Here's the drawing with two shaded views (mm, measured from the low corner). I have some questions. Round coordinates to 2 decimals unless told otherwise and drop trailing zeros. Write each loop counter-clockwise with the first axis right and the second up, starting at its lowest first coordinate (ties: lowest second). Pieces come first, ordered by that corner, then holes. Notation, with made-up numbers: M -26.75,36 L 17.25,36 A17 cw 17.25,58 Z; hole C -40,88.25 d10. An arc over 180 degrees is marked long. Write item = value, one per line. Start each with the question number.
(1) I want a section at A-A (y = 165). List the corners of the cut face in (x, z) for me, and give its area (3 significant figures).
(2) Will these pins go through, and if not, where does the flat tip stop? pin 1 Ø14.5 at (x, y) = (121, 165) entering from -Z; pin 2 Ø3 at (x, z) = (112.5, 4) entering from +Y; pin 3 Ø3 at (y, z) = (51.5, 3.5) entering from +X.
(3) I want a section at B-B (x = 91.5). List the corners of the cut face in (y, z) for me.
(4) I want a section at D-D (x = 121). List the corners of the cut face in (y, z) for me.
(5) I want a section at C-C (z = 1.9). List the corners of the cut face in (x, y) for me.
(6) I need wall thicknesses on line 1 along X through (y, z) = (225, 2.1); line 2 along Y through (x, z) = (121, 4.4); line 3 along Y through (x, z) = (72.5, 2.2). Which ranges of each line are inside material? Lowest first, please.
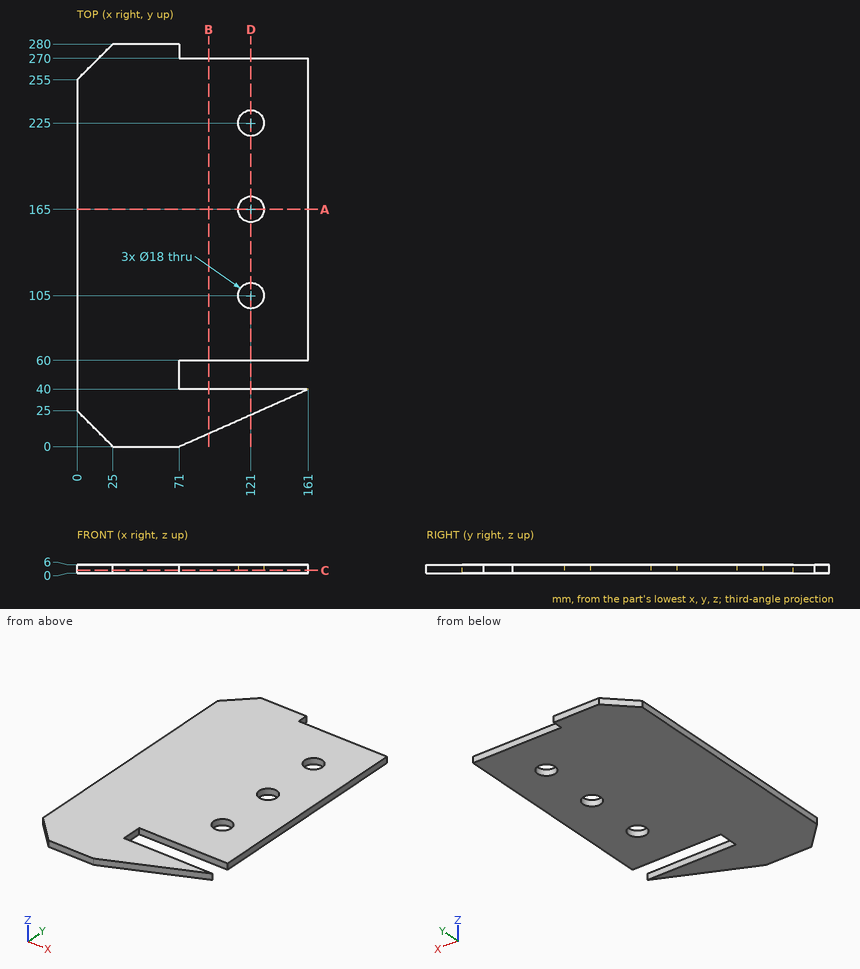
Returned:
q1.outline = M 0,0 L 112,0 L 112,6 L 0,6 Z; M 130,0 L 161,0 L 161,6 L 130,6 Z
q1.area = 858 mm²
q2.pin_1 = through
q2.pin_2 = 270
q2.pin_3 = 71
q3.outline = M 9.11,0 L 40,0 L 40,6 L 9.11,6 Z; M 60,0 L 270,0 L 270,6 L 60,6 Z
q4.outline = M 22.22,0 L 40,0 L 40,6 L 22.22,6 Z; M 60,0 L 96,0 L 96,6 L 60,6 Z; M 114,0 L 156,0 L 156,6 L 114,6 Z; M 174,0 L 216,0 L 216,6 L 174,6 Z; M 234,0 L 270,0 L 270,6 L 234,6 Z
q5.outline = M 0,25 L 25,0 L 71,0 L 161,40 L 71,40 L 71,60 L 161,60 L 161,270 L 71,270 L 71,280 L 25,280 L 0,255 Z; hole C 121,105 d18; hole C 121,165 d18; hole C 121,225 d18
q6.line_1 = 0 to 112, 130 to 161
q6.line_2 = 22.22 to 40, 60 to 96, 114 to 156, 174 to 216, 234 to 270
q6.line_3 = 0.67 to 40, 60 to 270
